```python
from build123d import *

# Parameters (mm, degrees)
SKETCH_R        = 16
PAD_DEPTH       = 6
SKETCH001_R     = 15.5
PAD001_DEPTH    = 1
SKETCH002_R     = 16
PAD002_DEPTH    = 6
SKETCH003_R     = 13.15
POCKET_DEPTH    = 6
SKETCH004_R     = 13.15
POCKET001_DEPTH = 6
SKETCH005_R     = 12
POCKET002_DEPTH = 1
SKETCH006_W     = 6
SKETCH006_H     = 10
POCKET003_DEPTH = 13


with BuildPart() as part:
    # Sketch → Pad (new body)
    with BuildSketch(Plane.XY):
        Circle(SKETCH_R)
    extrude(amount=PAD_DEPTH)

    # Sketch001 (on Face3 of Pad) → Pad001 (join)
    with BuildSketch(Plane.XY.offset(6)):
        Circle(SKETCH001_R)
    extrude(amount=PAD001_DEPTH)

    # Sketch002 (on Face5 of Pad001) → Pad002 (join)
    with BuildSketch(Plane.XY.offset(7)):
        Circle(SKETCH002_R)
    extrude(amount=PAD002_DEPTH)

    # Sketch003 (on Face3 of Pad002) → Pocket (cut)
    with BuildSketch(Plane.XY.offset(13)):
        Circle(SKETCH003_R)
    extrude(amount=-POCKET_DEPTH, mode=Mode.SUBTRACT)

    # Sketch004 (on Face9 of Pocket) → Pocket001 (cut)
    with BuildSketch(Plane(origin=(0, 0, 0), x_dir=(1, 0, 0), z_dir=(0, 0, -1))):
        Circle(SKETCH004_R)
    extrude(amount=-POCKET001_DEPTH, mode=Mode.SUBTRACT)

    # Sketch005 (on Face11 of Pocket001) → Pocket002 (cut)
    with BuildSketch(Plane(origin=(0, 0, 6), x_dir=(1, 0, 0), z_dir=(0, 0, -1))):
        Circle(SKETCH005_R)
    extrude(amount=-POCKET002_DEPTH, mode=Mode.SUBTRACT)

    # Sketch006 (on Face10 of Pocket002) → Pocket003 (cut)
    with BuildSketch(Plane(origin=(0, 0, 0), x_dir=(1, 0, 0), z_dir=(0, 0, -1))):
        with Locations((-13, 0)):
            Rectangle(SKETCH006_W, SKETCH006_H)
    extrude(amount=-POCKET003_DEPTH, mode=Mode.SUBTRACT)


solid = part.part
```
Verification items for the finished model (mm, model axes). A direction names the side the tool comes from. Coordinates: 2 decimals unless noted, no trailing zeros. Write each loop counter-clockwise with the first axis right and the second up, starting at its lowest first coordinate (ties: lowest second). Pieces come first, ordered by that corner, then holes. Notation, with made-up numbers: M -16.75,33 L 4.25,33 A30 ccw 4.25,72 Z; hole C 39.5,77 d10. An arc over 180 degrees is marked long. Answer as a JSON object with one key per item and string values. Group by question number.
(1) Gauge pin test, flat ends, axial feed: pin 1 (3.5 mm diameter, centred on x = -13.5, z = 6.5, fed in from +Y); pin 2 (5 mm diameter, centred on x = 4.5, z = 11.5, fed in from -Y); pin 3 (2 mm diameter, centred on x = 6.5, z = 5, fed in from -Y) (3 decimals); pin 4 (15.5 mm diameter, centred on x = -0.5, y = 3.5, fed in from -Z). Record the tip position at first contact, or that the pin passes through.
(2) Cross-section at A-A, the plane x = 0. Record the cut outline in (y, z).
(3) Release check for a two-part mould opening along Y. For faces 5 (the face through (15.987, -0.632, 2.958)), 6 (the face through (12, -6, 13)), 7 (the face through (12, 3, 6)) record: +Y half, -Y half, draft (parallel to the pull), parting line (faces both ways), or undercut.
(4) Cross-section at C-C, the plane z = 6.5. Record the cut outline in (x, y).
(5) Tool access check on faces 1 (the face through (2.6, 15.5, 7)), 2 (the face through (13.14, 0.51, 2.96)), 3 (the face through (12, -3, 7)), 4 (the face through (-14, 5, 6)). Record the directions out of +Z, -Z, +X, -X, +Y, -Y that give a thin tool (end or side, any length) a straight path to the whole face; none if there is none.
(6) Cross-section at D-D, the plane x = 6.5. Record the cut outline in (y, z).
(7) Cross-section at B-B, the plane y = 0. Record the cut outline in (x, z), and give its area (3 significant figures).
(8) Material ranges on line 1 (Y direction, x = 0, z = 6.75); line 2 (Z direction, x = 9, y = 8.5); line 3 (X direction, y = -10, z = 5.5), recorded low to high.
Reply:
{
 "1": {"pin 1": "y = 10.78", "pin 2": "y = -15.87", "pin 3": "y = -15.025", "pin 4": "through"},
 "2": {"outline": "M -16,0 L -13.15,0 L -13.15,6 L -12,6 L -12,7 L -13.15,7 L -13.15,13 L -16,13 L -16,7 L -15.5,7 L -15.5,6 L -16,6 Z; M 12,6 L 13.15,6 L 13.15,0 L 16,0 L 16,6 L 15.5,6 L 15.5,7 L 16,7 L 16,13 L 13.15,13 L 13.15,7 L 12,7 Z"},
 "3": {"face 5": "parting line", "face 6": "draft", "face 7": "undercut"},
 "4": {"outline": "M -14.67,-5 A15.5 ccw long -14.67,5 L -10.91,5 A12 cw long -10.91,-5 Z"},
 "5": {"face 1": "none", "face 2": "-Z", "face 3": "+Z", "face 4": "+Z, -Z, -X"},
 "6": {"outline": "M -14.62,0 L -11.43,0 L -11.43,6 L -10.09,6 L -10.09,7 L -11.43,7 L -11.43,13 L -14.62,13 L -14.62,7 L -14.07,7 L -14.07,6 L -14.62,6 Z; M 10.09,6 L 11.43,6 L 11.43,0 L 14.62,0 L 14.62,6 L 14.07,6 L 14.07,7 L 14.62,7 L 14.62,13 L 11.43,13 L 11.43,7 L 10.09,7 Z"},
 "7": {"outline": "M 12,6 L 13.15,6 L 13.15,0 L 16,0 L 16,6 L 15.5,6 L 15.5,7 L 16,7 L 16,13 L 13.15,13 L 13.15,7 L 12,7 Z", "area": "37.7 mm²"},
 "8": {"line 1": "-15.5 to -12, 12 to 15.5", "line 2": "6 to 7", "line 3": "-12.49 to -8.54, 8.54 to 12.49"}
}
